from build123d import *

# Parameters (mm, degrees)
SZKIC1_R                    = 10
SZKIC1_R_2                  = 3.3
DODANIE_WYCI_GNI_CIE1_DEPTH = 10
SZKIC2_R                    = 19
SZKIC2_R_2                  = 10
DODANIE_WYCI_GNI_CIE2_DEPTH = 38
SFAZOWANIE1_SIZE            = 0.5
SFAZOWANIE2_SIZE            = 0.5


with BuildPart() as part:
    # Szkic1 → Dodanie-wyciągnięcie1 (new body)
    with BuildSketch(Plane.XY):
        with BuildLine():
            Line((0, -22), (-18.894443628, -22))
            ThreePointArc((-18.894443628, -22), (-29, 0), (-18.894443628, 22))
            Line((-18.894443628, 22), (0, 22))
            Line((0, 22), (18.894443628, 22))
            ThreePointArc((18.894443628, 22), (29, 0), (18.894443628, -22))
            Line((18.894443628, -22), (0, -22))
        make_face()
        Circle(SZKIC1_R, mode=Mode.SUBTRACT)
        with Locations((-16.617009358, 16.617009358)):
            Circle(SZKIC1_R_2, mode=Mode.SUBTRACT)
        with Locations((-23.5, 0)):
            Circle(SZKIC1_R_2, mode=Mode.SUBTRACT)
        with Locations((-16.617009358, -16.617009358)):
            Circle(SZKIC1_R_2, mode=Mode.SUBTRACT)
        with Locations((16.617009358, -16.617009358)):
            Circle(SZKIC1_R_2, mode=Mode.SUBTRACT)
        with Locations((23.5, 0)):
            Circle(SZKIC1_R_2, mode=Mode.SUBTRACT)
        with Locations((16.617009358, 16.617009358)):
            Circle(SZKIC1_R_2, mode=Mode.SUBTRACT)
    extrude(amount=DODANIE_WYCI_GNI_CIE1_DEPTH)

    # Szkic2 → Dodanie-wyciągnięcie2 (add)
    with BuildSketch(Plane(origin=(0, 0, 0), x_dir=(-1, 0, 0), z_dir=(0, 0, -1))):
        Circle(SZKIC2_R)
        Circle(SZKIC2_R_2, mode=Mode.SUBTRACT)
    extrude(amount=DODANIE_WYCI_GNI_CIE2_DEPTH)

    # Sfazowanie1
    sfazowanie1_edges = [part.edges().sort_by_distance(p)[0] for p in [
        (-19.917009358, 16.617009358, 0),
        (-19.917009358, 16.617009358, 10),
        (-26.8, 0, 0),
        (-26.8, 0, 10),
        (-19.917009358, -16.617009358, 0),
        (-19.917009358, -16.617009358, 10),
        (13.317009358, -16.617009358, 0),
        (13.317009358, -16.617009358, 10),
        (20.2, 0, 0),
        (20.2, 0, 10),
        (13.317009358, 16.617009358, 0),
        (13.317009358, 16.617009358, 10),
    ]]
    chamfer(sfazowanie1_edges, length=SFAZOWANIE1_SIZE)

    # Sfazowanie2
    sfazowanie2_edges = [part.edges().sort_by_distance(p)[0] for p in [
        (29, 0, 10),
        (-10, 0, 10),
        (-29, 0, 10),
        (19, 0, -38),
        (10, 0, -38),
        (29, 0, 0),
        (-29, 0, 0),
    ]]
    chamfer(sfazowanie2_edges, length=SFAZOWANIE2_SIZE)


solid = part.part
Could you check a few things on this model? Use its own coordinates, in mm. A direction names the side the tool comes from. Give positions to 0.01 mm unless a question says otherwise; leave off trailing zeros. Order: outer loops, then holes, each group sorted by start corner. A loop starts at its lowest first (then second) coordinate and runs counter-clockwise, first axis right, second up. Notation, with made-up numbers: (38.25, 77) -> (93.25, 77) arc R22 ccw to (93.25, 91) -> close; hole circle Ø4 at (-2, 88.5). An arc over 180 degrees is marked (long way). Return JSON: item names as keys, results as strings.
1. Thinking about a two-plate mould opening in X: for faces 3 (the flat face through (0, -22, 5)), 4 (the conical face through (28.633, 0.354, 9.865)), 5 (the cylindrical face through (19.765, -15.626, 4.937)), which applies, pulls with the +X half, pulls with the -X half, needs draft (parallel to the pull), parting line crosses it, or undercut?
Answer list:
{"face 3": "needs draft", "face 4": "pulls with the +X half", "face 5": "undercut"}
2. Imagine slicing it at A-A on x = 0. List the corners of the cut face in (y, z) for me.
Answer list:
{"outline": "(-22, 0) -> (-19, 0) -> (-19, -37.5) -> (-18.5, -38) -> (-10.5, -38) -> (-10, -37.5) -> (-10, 9.5) -> (-10.5, 10) -> (-22, 10) -> close; (10, -37.5) -> (10.5, -38) -> (18.5, -38) -> (19, -37.5) -> (19, 0) -> (22, 0) -> (22, 10) -> (10.5, 10) -> (10, 9.5) -> close"}
3. Imagine slicing it at C-C on z = 5. List the corners of the cut face in (x, y) for me.
Answer list:
{"outline": "(-18.89, -22) -> (18.89, -22) arc R29 ccw to (18.89, 22) -> (-18.89, 22) arc R29 ccw to start; hole circle Ø6.6 at (-23.5, 0); hole circle Ø6.6 at (-16.62, -16.62); hole circle Ø6.6 at (-16.62, 16.62); hole circle Ø20 at (0, 0); hole circle Ø6.6 at (16.62, -16.62); hole circle Ø6.6 at (16.62, 16.62); hole circle Ø6.6 at (23.5, 0)"}
4. I need wall thicknesses on line 1 (X direction, y = -2, z = 7.5); line 2 (X direction, y = -1, z = 6); line 3 (X direction, y = -2, z = -34.5). Which ranges of each line are inside material? Lowest first, please. Write a range as from..to.
Answer list:
{"line 1": "x = -28.93..-26.12, -20.88..-9.8, 9.8..20.88, 26.12..28.93", "line 2": "x = -28.98..-26.64, -20.36..-9.95, 9.95..20.36, 26.64..28.98", "line 3": "x = -18.89..-9.8, 9.8..18.89"}
5. Imagine slicing it at B-B on y = 0. Give the number of separate pieces and of enclosed holes in the cut face, then the cut area to 3 significant figures.
Answer list:
{"separate pieces": "4", "enclosed holes": "0", "area": "930 mm2"}
6. Imagine slicing it at D-D on z = -17.5. List the corners of the cut face in (x, y) for me.
Answer list:
{"outline": "circle Ø38 at (0, 0); hole circle Ø20 at (0, 0)"}
7. On a 3-axis mill with a long thin cutter (end or side, diameter ignored), from which of +Z, -Z, +X, -X, +Y, -Y can I reach the whole of each face in a straight line? I mean faces 1 (the cylindrical face through (-29, 0, 5)), 2 (the cylindrical face through (-8.767, -16.856, -18.488)). Say none if no direction works.
Answer list:
{"face 1": "+Z, -Z, -X", "face 2": "-Z"}
8. For pin 1 Ø4 at (x, z) = (5.5, -7.5) entering from -Y; pin 2 Ø1 at (x, z) = (16, -14.5) entering from -Y; pin 3 Ø2 at (y, z) = (17.5, -0.5) entering from -X, each with a flat end and sliding along its axis, tell me the tip position at first contact or that it passes through.
Answer list:
{"pin 1": "stops at y = -18.67", "pin 2": "stops at y = -10.99", "pin 3": "stops at x = -23.33"}
